Drawing for the job (mm, zero at the part's lowest x, y, z). Round coordinates to 2 decimals unless told otherwise and drop trailing zeros. Loops run counter-clockwise (first coordinate to the right, second up) from the corner with the lowest first, then second, coordinate; pieces in that order, holes last. Notation, with made-up numbers: M 19,89.25 L 62,89.25 A26 ccw 62,105.25 Z; hole C -28,87 d9. An arc over 180 degrees is marked long. Use a Markdown table: item, result. Add a question column.
Q1. Pin check, flat tip, straight feed: pin 1 (2.5 mm diameter, centred on x = 57.5, z = 7.5, fed in from +Y). Stop position of the tip, or through.
Q2. Probe line 1 (X direction, y = 2.3, z = 7.5); line 2 (X direction, y = 0.95, z = 7.5); line 3 (X direction, y = 1.9, z = 9.25). List the from-to ranges inside material, lowest first. Write a range as from..to.
Q3. Mould opens along X. For the marked faces 1 and 2 say: +X half, -X half, draft (parallel to the pull), parting line (faces both ways), or undercut.
Q4. Cut at A-A (y = 2.8). Give the cut face in (x, z), plus the area to 3 significant figures.
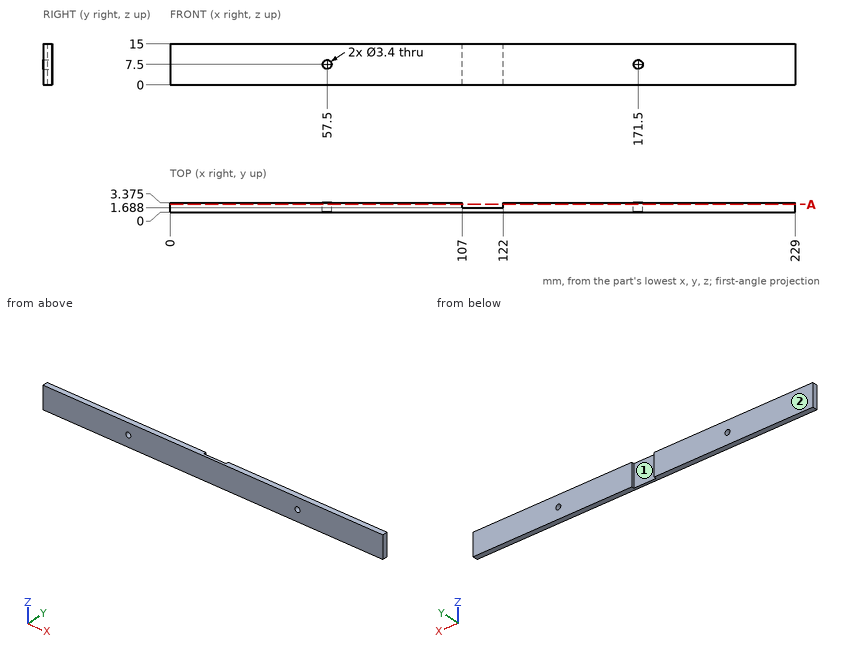
Checked values:
| question | item | result |
|---|---|---|
| 1 | pin 1 | passes through |
| 2 | line 1 | x = 0..55.8, 59.2..107, 122..169.8, 173.2..229 |
| 2 | line 2 | x = 0..55.8, 59.2..169.8, 173.2..229 |
| 2 | line 3 | x = 0..107, 122..229 |
| 3 | face 1 | undercut |
| 3 | face 2 | draft |
| 4 | outline | M 0,0 L 107,0 L 107,15 L 0,15 Z; M 122,0 L 229,0 L 229,15 L 122,15 Z; hole C 57.5,7.5 d3.4; hole C 171.5,7.5 d3.4 |
| 4 | area | 3,190 mm^2 |
